Design review of the part built by this model. Coordinates are the model's own, in mm. Face numbers are marked on the shaded views. A direction names the side the tool comes from. Coordinates: 2 decimals unless noted, no trailing zeros. Loops run counter-clockwise (first coordinate to the right, second up) from the corner with the lowest first, then second, coordinate; pieces in that order, holes last. Notation, with made-up numbers: (7.25, 87) - (45.25, 87) arc R24 ccw to (45.25, 118) - close; hole circle Ø10 at (67, -19). An arc over 180 degrees is marked (long way). Answer in a Markdown table with one row per item. Add a question column.
(1) We need section C-C, the plane x = 0. Write out the cut boundary in (y, z).
(2) Clearance check with flat-ended pins moving along their axes: pin 1 (6.5 mm diameter, centred on x = 0.5, z = 7.5, fed in from -Y); pin 2 (6 mm diameter, centred on x = 9.5, y = -2.5, fed in from +Z); pin 3 (1 mm diameter, centred on y = -13, z = 12.5, fed in from -X); pin 4 (5.5 mm diameter, centred on x = -2.5, y = -20.5, fed in from -Z). State where each tip first meets the part, or that it passes through.
(3) We need section B-B, the plane z = 5.5. Write out the cut boundary in (x, y).
(4) We need section A-A, the plane y = -13.5. Write out the cut boundary in (x, z), plus the area to 3 significant figures.
(5) To check wall thickness, follow L1, parallel to Y at x = 0, z = 7.35; L2, parallel to Y at x = 0, z = 3.75; L3, parallel to Z at x = 0, y = -16.2. State the ranges of each line that lie inside material, in increasing order. Write a range as [from, to].
(6) We need section D-D, the plane z = 8.75. Write out the cut boundary in (x, y).
(7) For the marked faces 1, 2, 3 and 4, list the 3-axis set-ups (+Z, -Z, +X, -X, +Y, -Y) from which the entire face can be reached by the end or side of a thin tool; tool diameter is ignored.
(8) The part is to be moulded in two halves that separate along X. For the marked faces 5, 6, 7 and 8, say which applies: released by +X, released by -X, zero draft, split by the parting line, or undercut.
from build123d import *

# Parameters (mm, degrees)
F1_DEPTH  = 16
F2_R      = 12.7
F3_DEPTH  = 8
F4_R      = 1.2
F5_R      = 3
F6_R      = 11.7
F7_DEPTH  = 1
F8_R      = 7.7
F9_DEPTH  = 6.4
F10_W     = 13
F10_H     = 13
F11_DEPTH = 6.8
F12_R     = 4.2
F13_DEPTH = 5.2


with BuildPart() as f1:
    # F0 (on Top) → F1 (new body)
    with BuildSketch(Plane.XY):
        with BuildLine():
            ThreePointArc((8, -9.6046863561), (11.3192314227, -5.3033008589), (12.5, 0))
            ThreePointArc((12.5, 0), (-5.3033008589, 11.3192314227), (-8, -9.6046863561))
            Line((-8, -9.6046863561), (-8, 0))
            Line((-8, 0), (8, 0))
            Line((8, 0), (8, -9.6046863561))
        make_face()
        with BuildLine():
            Line((-8, 0), (-8, -9.6046863561))
            ThreePointArc((-8, -9.6046863561), (0, -12.5), (8, -9.6046863561))
            Line((8, -9.6046863561), (8, 0))
            Line((8, 0), (-8, 0))
        make_face()
        with BuildLine():
            ThreePointArc((8, -9.6046863561), (0, -12.5), (-8, -9.6046863561))
            Line((-8, -9.6046863561), (-8, -25))
            Line((-8, -25), (8, -25))
            Line((8, -25), (8, -9.6046863561))
        make_face()
    extrude(amount=F1_DEPTH)

    # F2 (on face) → F3 (cut)
    with BuildSketch(Plane.XY.offset(16)):
        Circle(F2_R)
    extrude(amount=-F3_DEPTH, mode=Mode.SUBTRACT)

    # F4
    f4_edges = [f1.edges().sort_by_distance(p)[0] for p in [
        (-8, -9.863569, 12),
        (8, -9.863569, 12),
    ]]
    fillet(f4_edges, radius=F4_R)

    # F5
    f5_edges = [f1.edges().sort_by_distance(p)[0] for p in [
        (8, -9.604686, 4),
        (-8, -9.604686, 4),
    ]]
    fillet(f5_edges, radius=F5_R)

    # F6 (on face) → F7 (cut)
    with BuildSketch(Plane.XY.offset(8)):
        Circle(F6_R)
    extrude(amount=-F7_DEPTH, mode=Mode.SUBTRACT)

    # F8 (on face) → F9 (cut)
    with BuildSketch(Plane.XY.offset(7)):
        Circle(F8_R)
    extrude(amount=-F9_DEPTH, mode=Mode.SUBTRACT)

    # F10 (on face) → F11 (cut)
    with BuildSketch(Plane.XZ.offset(25)):
        with Locations((0, 8)):
            Rectangle(F10_W, F10_H)
    extrude(amount=-F11_DEPTH, mode=Mode.SUBTRACT)

    # F12 (on face) → F13 (cut)
    with BuildSketch(Plane.XZ.offset(18.2)):
        with Locations((0, 8)):
            Circle(F12_R)
    extrude(amount=-F13_DEPTH, mode=Mode.SUBTRACT)


solid = f1.part
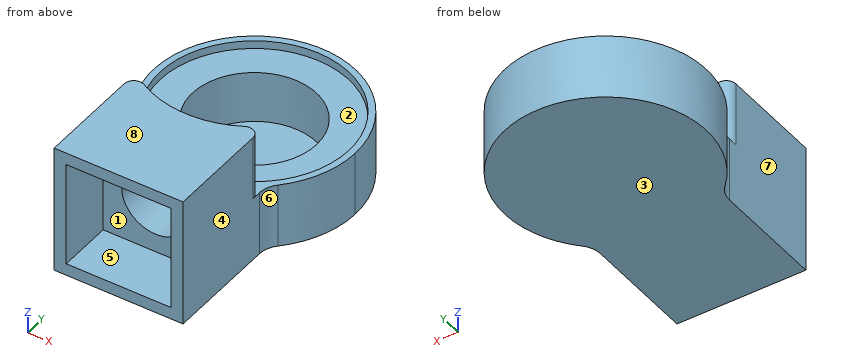
Responses:
| question | item | result |
|---|---|---|
| 1 | outline | (-25, 0) - (12.5, 0) - (12.5, 8) - (11.7, 8) - (11.7, 7) - (7.7, 7) - (7.7, 0.6) - (-7.7, 0.6) - (-7.7, 7) - (-11.7, 7) - (-11.7, 8) - (-12.7, 8) - (-12.7, 16) - (-25, 16) - (-25, 14.5) - (-18.2, 14.5) - (-18.2, 12.2) - (-13, 12.2) - (-13, 3.8) - (-18.2, 3.8) - (-18.2, 1.5) - (-25, 1.5) - close |
| 2 | pin 1 | stops at y = -13 |
| 2 | pin 2 | stops at z = 8 |
| 2 | pin 3 | stops at x = -8 |
| 2 | pin 4 | stops at z = 0 |
| 3 | outline | (-8.87, -8.81) arc R3 cw to (-8, -10.92) - (-8, -25) - (-6.5, -25) - (-6.5, -18.2) - (-3.37, -18.2) - (-3.37, -13) - (3.37, -13) - (3.37, -18.2) - (6.5, -18.2) - (6.5, -25) - (8, -25) - (8, -10.92) arc R3 cw to (8.87, -8.81) arc R12.5 ccw (long way) to start; hole circle Ø15.4 at (0, 0) |
| 4 | outline | (-8, 0) - (8, 0) - (8, 16) - (-8, 16) - close; hole circle Ø8.4 at (0, 8) |
| 4 | area | 201 mm2 |
| 5 | L1 | y = [-13, -11.7], [11.7, 12.5] |
| 5 | L2 | y = [-18.2, -7.7], [7.7, 12.5] |
| 5 | L3 | z = [0, 3.8], [12.2, 16] |
| 6 | outline | (-8, -25) - (-6.5, -25) - (-6.5, -18.2) - (-4.13, -18.2) - (-4.13, -13) - (4.13, -13) - (4.13, -18.2) - (6.5, -18.2) - (6.5, -25) - (8, -25) - (8, -12.12) arc R1.2 ccw to (6.21, -11.08) arc R12.7 cw to (-6.21, -11.08) arc R1.2 ccw to (-8, -12.12) - close |
| 7 | face 1 | -Y |
| 7 | face 2 | +Z |
| 7 | face 3 | -Z, +X, -X, +Y, -Y |
| 7 | face 4 | +Z, -Z, +X, -Y |
| 8 | face 5 | undercut |
| 8 | face 6 | released by +X |
| 8 | face 7 | released by -X |
| 8 | face 8 | zero draft |
